```python
from build123d import *

# Parameters (mm, degrees)
SKETCH_1_R               = 156
EXTRUDE_1_DEPTH          = 8
SKETCH_4_R               = 6
CUT_EXTRUDE_3_DEPTH      = 10
PATTERN_CIRCULAR_2_COUNT = 4
FILLET_1_R               = 0.3
SKETCH_8_R               = 8
CUT_EXTRUDE_7_DEPTH      = 10
PATTERN_CIRCULAR_3_COUNT = 2
SKETCH_9_R               = 8
CUT_EXTRUDE_8_DEPTH      = 10
SKETCH_10_R              = 2
CUT_EXTRUDE_9_DEPTH      = 10
PATTERN_CIRCULAR_5_COUNT = 4


with BuildPart() as part:
    # 草图1 → 凸台-拉伸1 (new body)
    with BuildSketch(Plane(origin=(0, 0, 0), x_dir=(0, 0, -1), z_dir=(1, 0, 0))):
        Circle(SKETCH_1_R)
    extrude(amount=EXTRUDE_1_DEPTH)

    # 草图4 → 切除-拉伸3 (cut)
    with BuildSketch(Plane(origin=(8, 0, 0), x_dir=(0, 0, -1), z_dir=(1, 0, 0))):
        with Locations((91.923881554, 91.923881554)):
            Circle(SKETCH_4_R)
    cut_extrude_3 = extrude(amount=-CUT_EXTRUDE_3_DEPTH, mode=Mode.SUBTRACT)

    # 阵列(圆周)2: 切除-拉伸3 ×4 about axis
    pattern_circular_2_axis = Axis((0, 0, 0), (1, 0, 0))
    for i in range(1, PATTERN_CIRCULAR_2_COUNT):
        add(cut_extrude_3.rotate(pattern_circular_2_axis, i * 360 / PATTERN_CIRCULAR_2_COUNT), mode=Mode.SUBTRACT)

    # 圆角1
    fillet_1_edges = [part.edges().sort_by_distance(p)[0] for p in [
        (0, 0, 156),
        (8, 0, 156),
    ]]
    fillet(fillet_1_edges, radius=FILLET_1_R)

    # 草图8 → 切除-拉伸7 (cut)
    with BuildSketch(Plane(origin=(8, 0, 0), x_dir=(0, 0, -1), z_dir=(1, 0, 0))):
        with Locations((42.426406871, -42.426406871)):
            Circle(SKETCH_8_R)
    cut_extrude_7 = extrude(amount=-CUT_EXTRUDE_7_DEPTH, mode=Mode.SUBTRACT)

    # 阵列(圆周)3: 切除-拉伸7 ×2 about axis
    pattern_circular_3_axis = Axis((0, 0, 0), (1, 0, 0))
    for i in range(1, PATTERN_CIRCULAR_3_COUNT):
        add(cut_extrude_7.rotate(pattern_circular_3_axis, i * 360 / PATTERN_CIRCULAR_3_COUNT), mode=Mode.SUBTRACT)

    # 草图9 → 切除-拉伸8 (cut)
    with BuildSketch(Plane(origin=(8, 0, 0), x_dir=(0, 0, -1), z_dir=(1, 0, 0))):
        Circle(SKETCH_9_R)
    extrude(amount=-CUT_EXTRUDE_8_DEPTH, mode=Mode.SUBTRACT)

    # 草图10 → 切除-拉伸9 (cut)
    with BuildSketch(Plane(origin=(8, 0, 0), x_dir=(0, 0, -1), z_dir=(1, 0, 0))):
        with Locations((36, 0)):
            Circle(SKETCH_10_R)
    cut_extrude_9 = extrude(amount=-CUT_EXTRUDE_9_DEPTH, mode=Mode.SUBTRACT)

    # 阵列(圆周)5: 切除-拉伸9 ×4 about axis
    pattern_circular_5_axis = Axis((0, 0, 0), (1, 0, 0))
    for i in range(1, PATTERN_CIRCULAR_5_COUNT):
        add(cut_extrude_9.rotate(pattern_circular_5_axis, i * 360 / PATTERN_CIRCULAR_5_COUNT), mode=Mode.SUBTRACT)


solid = part.part
```
Geometry check sheet. Reference: the model listing, model coordinates, mm. Give positions to 0.01 mm unless a question says otherwise; leave off trailing zeros.
1) Section check A-A, the plane x = 5.25. State how many separate pieces and enclosed holes the cut face has, and give its area (3 significant figures).
2) Material ranges on L1, parallel to Y at x = 4, z = -36; L2, parallel to Y at x = 4.25, z = 96; L3, parallel to Y at x = 2.75, z = -10.5, recorded low to high.
3) Gauge pin test, flat ends, axial feed: pin 1 (11 mm diameter, centred on y = 91.92, z = 91.92, fed in from -X); pin 2 (1 mm diameter, centred on x = 4.5, y = 88.5, fed in from -Z); pin 3 (1.5 mm diameter, centred on x = 2, y = -77.5, fed in from +Z); pin 4 (4 mm diameter, centred on x = 5, y = 122, fed in from -Z). Record the tip position at first contact, or that the pin passes through.
4) Release check for a two-part mould opening along Z. For faces 1 (the flat face through (8, -32, 2)), 2 (the cylindrical face through (4.056, -91.143, -97.873)), 3 (the cylindrical face through (3.948, 154.672, 20.308)) record: pulls with the +Z half, pulls with the -Z half, needs draft (parallel to the pull), parting line crosses it, or undercut.
Computed:
1. separate pieces: 1
1. enclosed holes: 11
1. area: 75,300 mm2
2. L1: y = -151.79 to -47.19, -37.66 to -2, 2 to 151.79
2. L2: y = -122.96 to -96.33, -87.52 to 87.52, 96.33 to 122.96
2. L3: y = -155.65 to 155.65
3. pin 1: passes through
3. pin 2: stops at z = -128.81
3. pin 3: stops at z = 135.81
3. pin 4: stops at z = -99.68
4. face 1: needs draft
4. face 2: undercut
4. face 3: parting line crosses it
